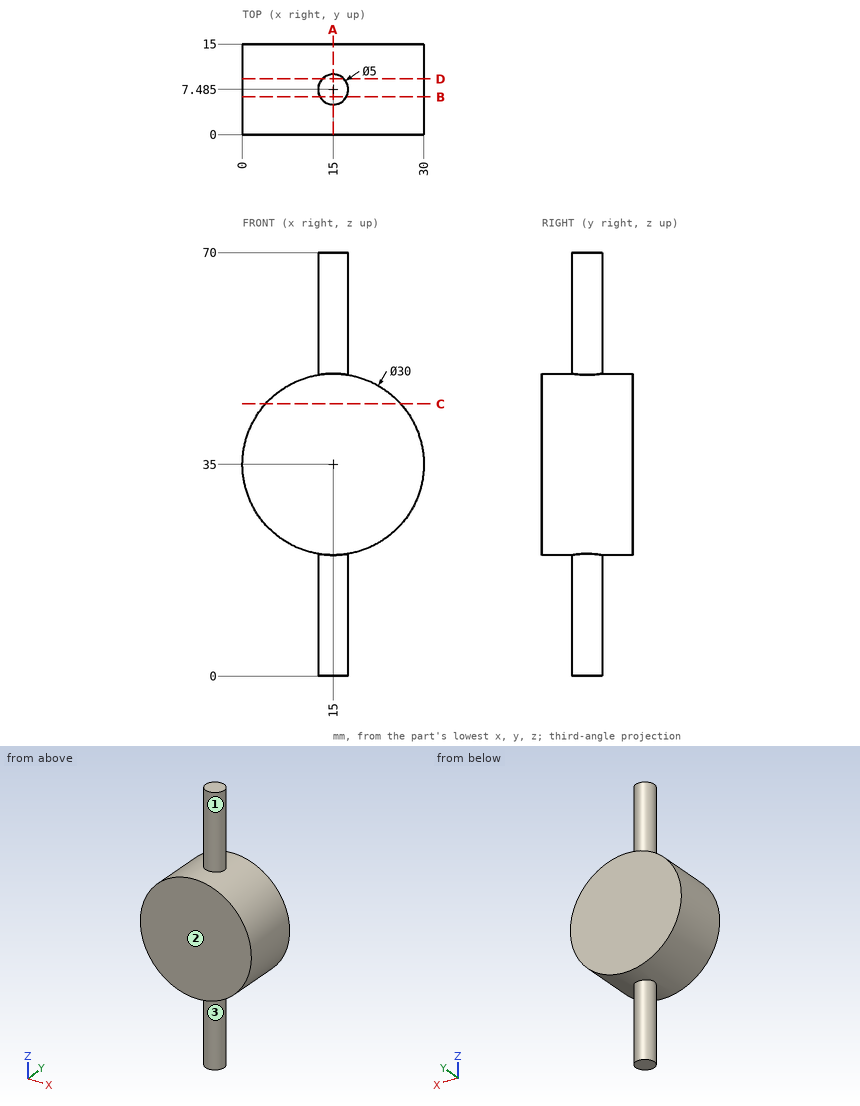
Source: three-view drawing plus pictorial views. Frame: mm from the lowest corner of the part. A direction names the side the tool comes from. Coordinates: 2 decimals unless noted, no trailing zeros. Order: outer loops, then holes, each group sorted by start corner. A loop starts at its lowest first (then second) coordinate and runs counter-clockwise, first axis right, second up. Notation, with made-up numbers: M -6.5,81.5 L 39.5,81.5 A17 ccw 39.5,98.5 Z; hole C -21,89 d1. An arc over 180 degrees is marked long. One line per question, with ' | ' between items. Start each with the question number.
Item 1: Ray query, probe 1 along Z at (x, y) = (17.5, 11); probe 2 along X at (y, z) = (8.5, 64) (1 decimal); probe 3 along Z at (x, y) = (11, 1.25). Return the intervals inside material, ascending. Write a range as [from, to].
Item 2: Cut plane B-B, the plane y = 6.25. Return the cut outline in (x, z).
Item 3: Cut plane A-A, the plane x = 15. Return the cut outline in (y, z) (1 decimal).
Item 4: Set-up query: the marked faces 1, 2 and 3. Return all of +Z, -Z, +X, -X, +Y, -Y with unobstructed straight access to the full face (end or side cutting, diameter ignored); none if empty.
Item 5: Pin query (flat end, axial travel): pin 1 Ø5 at (y, z) = (2.5, 28.5) entering from +X; pin 2 Ø5 at (x, y) = (4, 13.5) entering from -Z; pin 3 Ø3 at (x, z) = (16, 53.5) entering from -Y (1 decimal). Return the tip coordinate at first contact, or that it passes through.
Item 6: Cut plane C-C, the plane z = 45. Return the cut outline in (x, y).
Item 7: Cut plane D-D, the plane y = 9.25. Return the cut outline in (x, z) (1 decimal), then the cut area to 3 significant figures.
A:
1) probe 1: z = [20.21, 49.79] | probe 2: x = [12.7, 17.3] | probe 3: z = [20.54, 49.46]
2) outline: M 12.83,0 L 17.17,0 L 17.17,20.16 A15 ccw 17.17,49.84 L 17.17,70 L 12.83,70 L 12.83,49.84 A15 ccw 12.83,20.16 Z
3) outline: M 0,20 L 5,20 L 5,0 L 10,0 L 10,20 L 15,20 L 15,50 L 10,50 L 10,70 L 5,70 L 5,50 L 0,50 Z
4) face 1: +Z | face 2: +Z, -Z, +X, -X, -Y | face 3: -Z
5) pin 1: stops at x = 29.46 | pin 2: stops at z = 22.64 | pin 3: stops at y = 5
6) outline: M 3.82,0 L 26.18,0 L 26.18,15 L 3.82,15 Z
7) outline: M 13.2,0 L 16.8,0 L 16.8,20.1 A15 ccw 16.8,49.9 L 16.8,70 L 13.2,70 L 13.2,49.9 A15 ccw 13.2,20.1 Z | area: 849 mm2
